Could you check a few things on this model? Use its own coordinates, in mm. Face numbers are marked on the shaded views. Give positions to 0.01 mm unless a question says otherwise; leave off trailing zeros. Loops run counter-clockwise (first coordinate to the right, second up) from the corner with the lowest first, then second, coordinate; pieces in that order, holes last. Notation, with made-up numbers: (89, -15.5) -> (137, -15.5) arc R29 ccw to (137, 22.5) -> close; hole circle Ø8 at (58.25, 87). An arc over 180 degrees is marked (long way). Write item = value, one per line. Start each with the question number.
1) I need wall thicknesses on probe 1 along X at (y, z) = (42.5, 4.9); probe 2 along Y at (x, z) = (0, -61); probe 3 along X at (y, z) = (42.5, 5.5). Which ranges of each line are inside material? Lowest first, please. Write a range as from..to.
2) I want a section at B-B (z = -62). List the corners of the cut face in (x, y) for me, and give its area (3 significant figures).
3) If we mould it in two halves opening along Y, with no side actions, what happens to the marked faces 1, 2 and 3? For each: +Y half, -Y half, draft (parallel to the pull), parting line (faces both ways), or undercut.
4) I want a section at A-A (x = 0). List the corners of the cut face in (y, z) for me.
5) I'm going to push flat-ended pins straight in: pin 1 Ø1.2 at (x, y) = (-46.5, 65.5) entering from -Z; pin 2 Ø7.5 at (x, y) = (41, 67.5) entering from -Z; pin 3 Ø5 at (y, z) = (92.5, -10.5) entering from -X. Where does each tip first touch, or does it pass through?
from build123d import *

# Parameters (mm, degrees)
SKETCH1_R           = 49.9
SKETCH1_R_2         = 47.5
BOSS_EXTRUDE1_DEPTH = 100
BOSS_EXTRUDE2_START = 7
SKETCH2_R           = 49.9
SKETCH2_R_2         = 1.65
BOSS_EXTRUDE2_DEPTH = 7
SKETCH3_R           = 3.3
CUT_EXTRUDE1_DEPTH  = 3
CHAMFER1_SIZE       = 5
SKETCH5_R           = 3.3
CUT_EXTRUDE2_DEPTH  = 8


with BuildPart() as part:
    # Sketch1 → Boss-Extrude1 (new body)
    with BuildSketch(Plane.XY):
        with Locations((0, 55)):
            Circle(SKETCH1_R)
        with Locations((0, 55)):
            Circle(SKETCH1_R_2, mode=Mode.SUBTRACT)
    extrude(amount=-BOSS_EXTRUDE1_DEPTH)

    # Sketch2 → Boss-Extrude2 (add)
    with BuildSketch(Plane.XY.offset(BOSS_EXTRUDE2_START)):
        with Locations((0, 55)):
            Circle(SKETCH2_R)
        with Locations((41, 67.5)):
            Circle(SKETCH2_R_2, mode=Mode.SUBTRACT)
        with Locations((41, 42.5)):
            Circle(SKETCH2_R_2, mode=Mode.SUBTRACT)
        with Locations((-41, 67.5)):
            Circle(SKETCH2_R_2, mode=Mode.SUBTRACT)
        with Locations((-41, 42.5)):
            Circle(SKETCH2_R_2, mode=Mode.SUBTRACT)
    extrude(amount=-BOSS_EXTRUDE2_DEPTH)

    # Sketch3 → Cut-Extrude1 (cut)
    with BuildSketch(Plane.XY.offset(7)):
        with Locations((-41, 67.5)):
            Circle(SKETCH3_R)
        with Locations((-41, 42.5)):
            Circle(SKETCH3_R)
        with Locations((41, 67.5)):
            Circle(SKETCH3_R)
        with Locations((41, 42.5)):
            Circle(SKETCH3_R)
    extrude(amount=-CUT_EXTRUDE1_DEPTH, mode=Mode.SUBTRACT)

    # Chamfer1
    # the kernel refuses this chamfer: 5 mm, written as the material it takes off along each edge
    with BuildSketch(Plane(origin=(0, 55, 7), x_dir=(1, 0, 0), z_dir=(0, -1, 0))) as chamfer1_piece_1:
        Polygon((49.9, -CHAMFER1_SIZE), (49.9 - CHAMFER1_SIZE, 0), (49.9, 0), align=None)
    revolve(axis=Axis((0, 55, 7), (0, 0, 1)), mode=Mode.SUBTRACT)

    # Sketch4 → Cut-Revolve1 (revolve, cut)
    with BuildSketch(Plane(origin=(0, 0, 0), x_dir=(0, 0, -1), z_dir=(1, 0, 0)), mode=Mode.PRIVATE) as cut_revolve1_sk:
        Polygon((13, 104.9), (14, 103.9), (87.5, 103.9), (88.5, 104.9), align=None)
    revolve(cut_revolve1_sk.sketch.rotate(Axis((0, 55, 2), (0, 0, 1)), 76.43618314), axis=Axis((0, 55, 2), (0, 0, 1)), mode=Mode.SUBTRACT)

    # Sketch5 → Cut-Extrude2 (cut)
    with BuildSketch(Plane(origin=(0, 0, -100), x_dir=(-1, 0, 0), z_dir=(0, 0, -1))):
        with Locations((-44, 45)):
            Circle(SKETCH5_R)
        with Locations((-44, 65)):
            Circle(SKETCH5_R)
        with Locations((44, 45)):
            Circle(SKETCH5_R)
        with Locations((44, 65)):
            Circle(SKETCH5_R)
    extrude(amount=-CUT_EXTRUDE2_DEPTH, mode=Mode.SUBTRACT)


solid = part.part
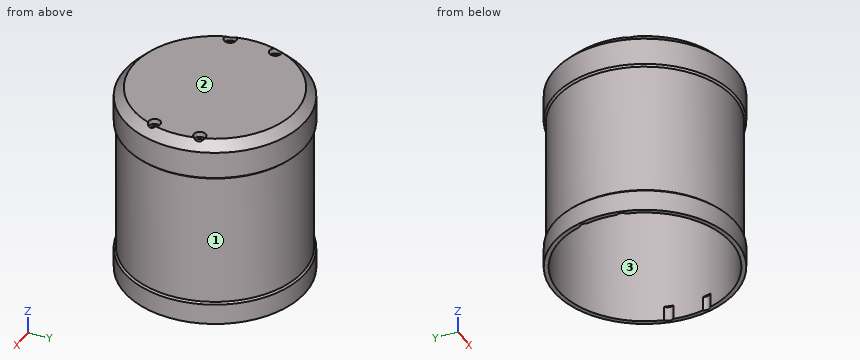
Answer list:
q1.probe_1 = -45.31..-44.3, -37.7..37.7, 44.3..45.31
q1.probe_2 = 6.1..7.5, 102.5..103.9
q1.probe_3 = -44.68..-44.3, -37.7..37.7, 44.3..44.68
q2.outline = circle Ø97.8 at (0, 55); hole circle Ø95 at (0, 55)
q2.area = 424 mm^2
q3.face_1 = parting line
q3.face_2 = draft
q3.face_3 = undercut
q4.outline = (5.1, -100) -> (7.5, -100) -> (7.5, 0) -> (102.5, 0) -> (102.5, -100) -> (104.9, -100) -> (104.9, -88.5) -> (103.9, -87.5) -> (103.9, -14) -> (104.9, -13) -> (104.9, 2) -> (99.9, 7) -> (10.1, 7) -> (5.1, 2) -> (5.1, -13) -> (6.1, -14) -> (6.1, -87.5) -> (5.1, -88.5) -> close
q5.pin_1 = -92
q5.pin_2 = 0
q5.pin_3 = -35.57
